Source: CAD feature listing. Evaluate the final solid. Frame: model axes, mm. Round coordinates to 2 decimals unless told otherwise and drop trailing zeros. Order: outer loops, then holes, each group sorted by start corner. A loop starts at its lowest first (then second) coordinate and runs counter-clockwise, first axis right, second up. Notation, with made-up numbers: (-1, 80) - (16, 80) arc R27 ccw to (16, 109) - close; hole circle Ø3 at (5.5, -39.5). An arc over 180 degrees is marked (long way). Return JSON: item names as keys, results as strings. Group by question number.
1) Section B-B, the plane x = -29. Return loops of the section in (y, z) (3 decimals), plus the area to 3 significant figures.
2) Section C-C, the plane y = 1.4. Return loops of the section in (x, z) (3 decimals).
3) Contact query for flat-ended pins moving along their axis: P1, Ø3.5, axis at x = 15, z = 0, coming from the +Y side; P2, Ø5, axis at x = 12.7, z = 0, coming from the +Y side. Output: stop coordinate, or through.
4) Ray query, line 1 (Z direction, x = 29, y = 3.65) (3 decimals); line 2 (Z direction, x = -12.7, y = 1.6); line 3 (X direction, y = 5.25, z = 4). Return the intervals inside material, ascending. Write a range as from..to.
5) Section A-A, the plane z = -24.5. Return loops of the section in (x, y) (3 decimals).
6) Section D-D, the plane x = 14. Return loops of the section in (y, z).
```python
from build123d import *

# Parameters (mm, degrees)
SKETCH2_W               = 80
SKETCH2_H               = 60
BOSS_EXTRUDE2_DEPTH     = 6
SKETCH3_R               = 3.2
CUT_EXTRUDE1_DEPTH      = 6
CUT_EXTRUDE2_DEPTH      = 2
SKETCH6_R               = 1.375
CUT_EXTRUDE3_DEPTH      = 6
MIRROR4_COPY_1_SKETCH_R = 1.375
MIRROR4_COPY_1_DEPTH    = 6


with BuildPart() as part:
    # Sketch2 → Boss-Extrude2 (new body)
    with BuildSketch(Plane(origin=(0, 0, 0), x_dir=(1, 0, 0), z_dir=(0, 1, 0))):
        Rectangle(SKETCH2_W, SKETCH2_H)
    extrude(amount=BOSS_EXTRUDE2_DEPTH)

    # Sketch3 → Cut-Extrude1 (cut)
    with BuildSketch(Plane(origin=(0, 6, 0), x_dir=(1, 0, 0), z_dir=(0, 1, 0))):
        with Locations((-12.7, 0)):
            Circle(SKETCH3_R)
    cut_extrude1 = extrude(amount=-CUT_EXTRUDE1_DEPTH, mode=Mode.SUBTRACT)

    # Sketch5 → Cut-Extrude2 (cut)
    with BuildSketch(Plane(origin=(0, 6, 0), x_dir=(1, 0, 0), z_dir=(0, 1, 0))):
        Polygon((-9.409372911, -6.096865864), (-5.774645734, -0.198666278), (-9.065272823, 5.898199586), (-15.990627089, 6.096865864), (-19.625354266, 0.198666278), (-16.334727177, -5.898199586), align=None)
    cut_extrude2 = extrude(amount=-CUT_EXTRUDE2_DEPTH, mode=Mode.SUBTRACT)

    # Mirror2: Cut-Extrude1, Cut-Extrude2 across plane
    add(cut_extrude1.mirror(Plane(origin=(0, 0, 0), x_dir=(0, 0, 1), z_dir=(1, 0, 0))), mode=Mode.SUBTRACT)
    add(cut_extrude2.mirror(Plane(origin=(0, 0, 0), x_dir=(0, 0, 1), z_dir=(1, 0, 0))), mode=Mode.SUBTRACT)

    # Sketch6 → Cut-Extrude3 (cut)
    with BuildSketch(Plane(origin=(0, 6, 0), x_dir=(1, 0, 0), z_dir=(0, 1, 0))):
        with Locations((-29, 24.5)):
            Circle(SKETCH6_R)
    cut_extrude3 = extrude(amount=-CUT_EXTRUDE3_DEPTH, mode=Mode.SUBTRACT)

    # Mirror3: Cut-Extrude3 across plane
    add(cut_extrude3.mirror(Plane.XY), mode=Mode.SUBTRACT)

    # Mirror4: Cut-Extrude3 across plane
    add(cut_extrude3.mirror(Plane(origin=(0, 0, 0), x_dir=(0, 0, 1), z_dir=(1, 0, 0))), mode=Mode.SUBTRACT)

    # Mirror4 copy 1 sketch → Mirror4 copy 1 (cut)
    with BuildSketch(Plane(origin=(0, 6, 0), x_dir=(-1, 0, 0), z_dir=(0, 1, 0))):
        with Locations((-29, 24.5)):
            Circle(MIRROR4_COPY_1_SKETCH_R)
    extrude(amount=-MIRROR4_COPY_1_DEPTH, mode=Mode.SUBTRACT)


solid = part.part
```
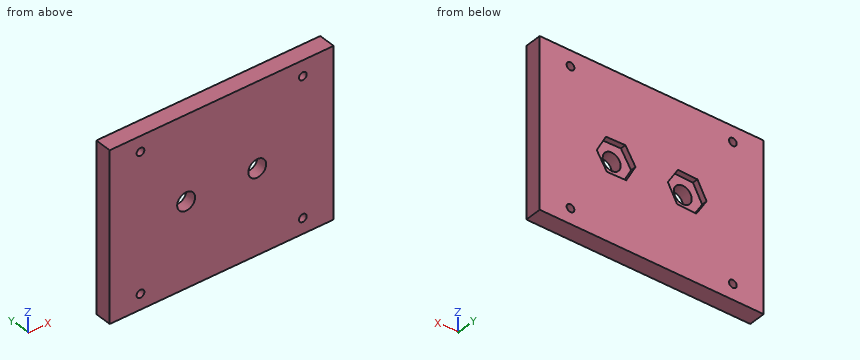
Geometry check:
{
 "1": {"outline": "(0, -30) - (6, -30) - (6, -25.875) - (0, -25.875) - close; (0, -23.125) - (6, -23.125) - (6, 23.125) - (0, 23.125) - close; (0, 25.875) - (6, 25.875) - (6, 30) - (0, 30) - close", "area": "327 mm2"},
 "2": {"outline": "(-40, -30) - (40, -30) - (40, 30) - (-40, 30) - close; hole circle Ø2.75 at (-29, -24.5); hole circle Ø2.75 at (-29, 24.5); hole circle Ø6.4 at (-12.7, 0); hole circle Ø6.4 at (12.7, 0); hole circle Ø2.75 at (29, -24.5); hole circle Ø2.75 at (29, 24.5)"},
 "3": {"P1": "y = 4", "P2": "through"},
 "4": {"line 1": "-30..-25.875, -23.125..23.125, 25.875..30", "line 2": "-30..-3.2, 3.2..30", "line 3": "-40..-17.36, -8.12..8.12, 17.36..40"},
 "5": {"outline": "(-40, 0) - (-30.375, 0) - (-30.375, 6) - (-40, 6) - close; (-27.625, 0) - (27.625, 0) - (27.625, 6) - (-27.625, 6) - close; (30.375, 0) - (40, 0) - (40, 6) - (30.375, 6) - close"},
 "6": {"outline": "(0, -30) - (6, -30) - (6, -6.04) - (4, -6.04) - (4, -2.92) - (0, -2.92) - close; (0, 2.92) - (4, 2.92) - (4, 5.97) - (6, 5.97) - (6, 30) - (0, 30) - close"}
}
